Verification items for the finished model (mm, model axes). A direction names the side the tool comes from. Coordinates: 2 decimals unless noted, no trailing zeros. Loops run counter-clockwise (first coordinate to the right, second up) from the corner with the lowest first, then second, coordinate; pieces in that order, holes last. Notation, with made-up numbers: (45, 10.25) -> (82, 10.25) arc R14 ccw to (82, 26.25) -> close; hole circle Ø4 at (-17.5, 31.5). An arc over 180 degrees is marked (long way). Write item = value, one per line.
```python
from build123d import *

# Parameters (mm, degrees)
SKETCH_1_W          = 32
SKETCH_1_H          = 19
SKETCH_1_R          = 1.6
EXTRUDE_1_DEPTH     = 1
SKETCH_3_W          = 32
SKETCH_3_H          = 4.75
EXTRUDE_2_DEPTH     = 2.8
SKETCH_4_W          = 32
SKETCH_4_H          = 1
EXTRUDE_3_DEPTH     = 2.8
EXTRUDE_4_DEPTH     = 2
EXTRUDE_5_DEPTH     = 7
CHAMFER_1_SIZE      = 7
SKETCH_7_R          = 1.6
EXTRUDE_6_DEPTH     = 1
SKETCH_8_W          = 4
SKETCH_8_H          = 16
CUT_EXTRUDE_1_DEPTH = 31.686967918
SKETCH_9_W          = 27
SKETCH_9_H          = 1.5
CUT_EXTRUDE_2_DEPTH = 1
SKETCH_10_W         = 3
SKETCH_10_H         = 19
CUT_EXTRUDE_3_DEPTH = 31.686967918
CHAMFER_2_SIZE      = 3


with BuildPart() as part:
    # 草图1 → 凸台-拉伸1 (new body)
    with BuildSketch(Plane(origin=(0, 0, 0), x_dir=(1, 0, 0), z_dir=(0, 1, 0))):
        with Locations((8.5, -5.5)):
            Rectangle(SKETCH_1_W, SKETCH_1_H)
        with Locations(Location((0, 0, 0), (0, 0, 270))):
            Circle(SKETCH_1_R, mode=Mode.SUBTRACT)
        with Locations(Location((17, 0, 0), (0, 0, 270))):
            Circle(SKETCH_1_R, mode=Mode.SUBTRACT)
    extrude(amount=EXTRUDE_1_DEPTH)

    # 草图3 → 凸台-拉伸2 (add)
    with BuildSketch(Plane(origin=(0, 1, 0), x_dir=(1, 0, 0), z_dir=(0, 1, 0))):
        with Locations((8.5, -11.525)):
            Rectangle(SKETCH_3_W, SKETCH_3_H)
    extrude(amount=EXTRUDE_2_DEPTH)

    # 草图4 → 凸台-拉伸3 (add)
    with BuildSketch(Plane(origin=(0, 1, 0), x_dir=(1, 0, 0), z_dir=(0, 1, 0))):
        with Locations((8.5, -7.4)):
            Rectangle(SKETCH_4_W, SKETCH_4_H)
    extrude(amount=EXTRUDE_3_DEPTH)

    # 草图5 → 凸台-拉伸4 (add)
    with BuildSketch(Plane(origin=(24.5, 0, 0), x_dir=(0, 0, -1), z_dir=(1, 0, 0))):
        Polygon((-15, 0), (4, 0), (4, 1), (-6.9, 1), (-6.9, 3.8), (-7.9, 3.8), (-7.9, 1), (-9.15, 1), (-9.15, 3.8), (-13.9, 3.8), (-13.9, 1), (-15, 1), align=None)
    extrude(amount=EXTRUDE_4_DEPTH)

    # 草图6 → 凸台-拉伸5 (add)
    with BuildSketch(Plane.ZY.offset(7.5)):
        Polygon((-4, 0), (15, 0), (15, 1), (13.9, 1), (13.9, 3.8), (9.15, 3.8), (9.15, 1), (7.9, 1), (7.9, 3.8), (6.9, 3.8), (6.9, 1), (-4, 1), align=None)
    extrude(amount=EXTRUDE_5_DEPTH)

    # 倒角1
    chamfer_1_edges = [part.edges().sort_by_distance(p)[0] for p in [
        (26.5, 0.5, -4),
        (-14.5, 0.5, -4),
    ]]
    chamfer(chamfer_1_edges, length=CHAMFER_1_SIZE)

    # 草图7 → 凸台-拉伸6 (add)
    with BuildSketch(Plane(origin=(0, 1, 0), x_dir=(1, 0, 0), z_dir=(0, 1, 0))):
        Polygon((26.5, -6.9), (26.5, -3), (19.5, 4), (-7.5, 4), (-14.5, -3), (-14.5, -6.9), align=None)
        with Locations(Location((17, 0, 0), (0, 0, 270))):
            Circle(SKETCH_7_R, mode=Mode.SUBTRACT)
        with Locations(Location((0, 0, 0), (0, 0, 270))):
            Circle(SKETCH_7_R, mode=Mode.SUBTRACT)
    extrude(amount=EXTRUDE_6_DEPTH)

    # 草图8 → 切除-拉伸1 (cut, through all)
    with BuildSketch(Plane(origin=(0, 3.8, 0), x_dir=(1, 0, 0), z_dir=(0, 1, 0))):
        with Locations((-12.5, -7)):
            Rectangle(SKETCH_8_W, SKETCH_8_H)
    extrude(amount=-CUT_EXTRUDE_1_DEPTH, mode=Mode.SUBTRACT)

    # 草图9 → 切除-拉伸2 (cut)
    with BuildSketch(Plane(origin=(0, 2, 0), x_dir=(1, 0, 0), z_dir=(0, 1, 0))):
        with Locations((3, -6.15)):
            Rectangle(SKETCH_9_W, SKETCH_9_H)
    extrude(amount=-CUT_EXTRUDE_2_DEPTH, mode=Mode.SUBTRACT)

    # 草图10 → 切除-拉伸3 (cut, through all)
    with BuildSketch(Plane.XZ):
        with Locations((-9, 5.5)):
            Rectangle(SKETCH_10_W, SKETCH_10_H)
    extrude(amount=-CUT_EXTRUDE_3_DEPTH, mode=Mode.SUBTRACT)

    # 倒角2
    chamfer_2_edges = [part.edges().sort_by_distance(p)[0] for p in [
        (-7.5, 1, -4),
    ]]
    chamfer(chamfer_2_edges, length=CHAMFER_2_SIZE)


solid = part.part
```
1) Tool access check on faces 4 (the face through (10, 2, 13.9)), 5 (the face through (10, 2, 6.9)), 6 (the face through (10, 0, 5)), 7 (the face through (10, 1, 9)), 8 (the face through (10, 3.8, 12)). Record the directions out of +Z, -Z, +X, -X, +Y, -Y that give a thin tool (end or side, any length) a straight path to the whole face; none if there is none.
Ans:
face_4 = +Z, +X, -X, +Y
face_5 = -X, +Y
face_6 = +Z, -Z, +X, -X, -Y
face_7 = +X, -X, +Y
face_8 = +Z, -Z, +X, -X, +Y
2) Sectioned sample at B-B, the plane x = 0. Record the cut outline in (y, z).
Ans:
outline = (0, -4) -> (2, -4) -> (2, -1.6) -> (0, -1.6) -> close; (0, 1.6) -> (2, 1.6) -> (2, 5.4) -> (1, 5.4) -> (1, 6.9) -> (3.8, 6.9) -> (3.8, 7.9) -> (1, 7.9) -> (1, 9.15) -> (3.8, 9.15) -> (3.8, 13.9) -> (1, 13.9) -> (1, 15) -> (0, 15) -> close
3) Release check for a two-part mould opening along Z. For faces 1 (the face through (16.5, 1.5, 6.2)), 2 (the face through (23, 1, -0.5)), 3 (the face through (9.7, 1, 14.5)) record: pulls with the +Z half, pulls with the -Z half, needs draft (parallel to the pull), parting line crosses it, or undercut.
Ans:
face_1 = undercut
face_2 = pulls with the -Z half
face_3 = needs draft
4) Material ranges on line 1 (Z direction, x = 10, y = 1.6); line 2 (Z direction, x = 16, y = 2.3); line 3 (X direction, y = 0.9, z = 0), recorded low to high.
Ans:
line_1 = -4 to 5.4, 6.9 to 7.9, 9.15 to 13.9
line_2 = 6.9 to 7.9, 9.15 to 13.9
line_3 = -7.5 to -1.6, 1.6 to 15.4, 18.6 to 23.5
5) Depth check by flat-ended pin: pin 1 Ø0.5 at (y, z) = (1.5, 6) entering from -X; pin 2 Ø0.8 at (x, z) = (6, 6) entering from +Y; pin 3 Ø0.5 at (x, y) = (-1, 1.5) entering from +Z. Enter the tip coordinate at first touch or a pass-through.
Ans:
pin_1 = 16.5
pin_2 = 1
pin_3 = 13.9
6) Sectioned sample at D-D, the plane x = 24.5. Record the cut outline in (y, z).
Ans:
outline = (0, 1) -> (2, 1) -> (2, 6.9) -> (3.8, 6.9) -> (3.8, 7.9) -> (1, 7.9) -> (1, 9.15) -> (3.8, 9.15) -> (3.8, 13.9) -> (1, 13.9) -> (1, 15) -> (0, 15) -> close
7) Sectioned sample at A-A, the plane y = 1.4. Record the cut outline in (x, z), plus the area to 3 significant figures.
Ans:
outline = (-7.5, -1) -> (-4.5, -4) -> (19.5, -4) -> (26.5, 3) -> (26.5, 7.9) -> (-7.5, 7.9) -> (-7.5, 6.9) -> (16.5, 6.9) -> (16.5, 5.4) -> (-7.5, 5.4) -> close; (-7.5, 9.15) -> (26.5, 9.15) -> (26.5, 13.9) -> (-7.5, 13.9) -> close; hole circle Ø3.2 at (0, 0); hole circle Ø3.2 at (17, 0)
area = 485 mm2
8) Sectioned sample at C-C, the plane z = 0. Record the cut outline in (x, y), plus the area to 3 significant figures.
Ans:
outline = (-7.5, 0) -> (-1.6, 0) -> (-1.6, 2) -> (-7.5, 2) -> close; (1.6, 0) -> (15.4, 0) -> (15.4, 2) -> (1.6, 2) -> close; (18.6, 0) -> (23.5, 0) -> (23.5, 2) -> (18.6, 2) -> close
area = 49.2 mm2
